Could you check a few things on this model? Use its own coordinates, in mm. Face numbers are marked on the shaded views. A direction names the side the tool comes from. Coordinates: 2 decimals unless noted, no trailing zeros. Loops run counter-clockwise (first coordinate to the right, second up) from the corner with the lowest first, then second, coordinate; pieces in that order, holes last. Notation, with made-up numbers: (72.5, -21) -> (78.5, -21) arc R18 cw to (78.5, -4) -> close; hole circle Ø10 at (37.25, 71.25). An arc over 180 degrees is marked (long way). One line per question, with ' | ' between items.
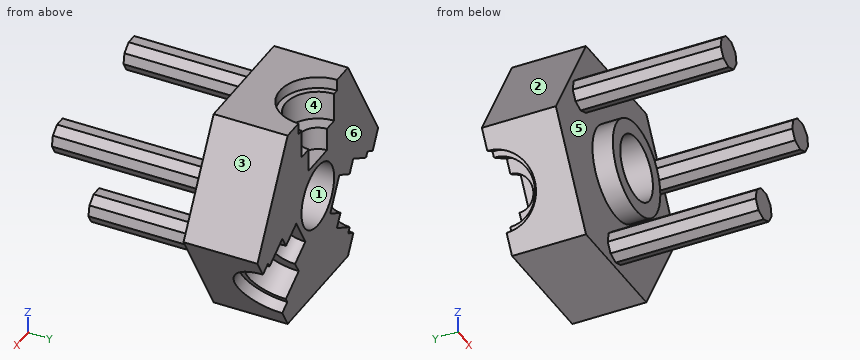
```python
from build123d import *

# Parameters (mm, degrees)
BOSS_EXTRUDE1_DEPTH = 12.7
SKETCH2_R           = 8
SKETCH2_R_2         = 5.5
BOSS_EXTRUDE2_DEPTH = 3.499999906
CIRPATTERN1_COUNT   = 3
SKETCH6_R           = 5.5
CUT_EXTRUDE1_DEPTH  = 17.199999906
BOSS_EXTRUDE3_DEPTH = 25.4


with BuildPart() as part:
    # Sketch1 → Boss-Extrude1 (new body)
    with BuildSketch(Plane(origin=(0, 0, 0), x_dir=(1, 0, 0), z_dir=(0, 1, 0))):
        Polygon((10.16, -17.597636205), (20.32, 0), (10.16, 17.597636205), (-10.16, 17.597636205), (-20.32, 0), (-10.16, -17.597636205), align=None)
    extrude(amount=BOSS_EXTRUDE1_DEPTH)

    # Sketch2 → Boss-Extrude2 (add)
    with BuildSketch(Plane.XZ):
        Circle(SKETCH2_R)
        Circle(SKETCH2_R_2, mode=Mode.SUBTRACT)
    extrude(amount=BOSS_EXTRUDE2_DEPTH)

    # Sketch5 → Cut-Revolve1 (revolve, cut)
    with BuildSketch(Plane(origin=(0, 12.7, 0), x_dir=(1, 0, 0), z_dir=(0, 1, 0))):
        Polygon((0, -17.597636205), (0, -6.597636205), (-3.065310501, -6.597636205), (-3.065310501, -10.597636205), (-5.5, -10.597636205), (-5.5, -15.597636205), (-6.5, -15.597636205), (-6.5, -17.597636205), align=None)
    cut_revolve1 = revolve(axis=Axis((0, 12.7, 17.597636205), (0, 0, -1)), mode=Mode.SUBTRACT)

    # CirPattern1: Cut-Revolve1 ×3 about axis
    cirpattern1_axis = Axis((0, 0, 0), (0, 1, 0))
    for i in range(1, CIRPATTERN1_COUNT):
        add(cut_revolve1.rotate(cirpattern1_axis, i * 360 / CIRPATTERN1_COUNT), mode=Mode.SUBTRACT)

    # Sketch6 → Cut-Extrude1 (cut, through all)
    with BuildSketch(Plane(origin=(0, 12.7, 0), x_dir=(1, 0, 0), z_dir=(0, 1, 0))):
        Circle(SKETCH6_R)
    extrude(amount=-CUT_EXTRUDE1_DEPTH, mode=Mode.SUBTRACT)

    # Sketch8 → Boss-Extrude3 (add)
    with BuildSketch(Plane(origin=(0, 0, 0), x_dir=(1, 0, 0), z_dir=(0, 1, 0))):
        Polygon((-1.915248015, 16.000954519), (-2.83973241, 14.399700576), (-2.518662349, 12.578821777), (-1.102270082, 11.390327548), (0.746698708, 11.390327548), (2.163090976, 12.578821777), (2.484161036, 14.399700576), (1.559676641, 16.000954519), (-0.177785687, 16.63333909), align=None)
        Polygon((14.814348451, -6.342126208), (13.889864056, -4.740872265), (12.152401728, -4.108487694), (10.4149394, -4.740872265), (9.490455005, -6.342126208), (9.811525066, -8.163005007), (11.227917333, -9.351499236), (13.076886123, -9.351499236), (14.49327839, -8.163005007), align=None)
        Polygon((-12.90012529, -9.658841379), (-11.0511565, -9.658841379), (-9.634764233, -8.47034715), (-9.313694172, -6.64946835), (-10.238178567, -5.048214407), (-11.975640895, -4.415829837), (-13.713103223, -5.048214407), (-14.637587618, -6.64946835), (-14.316517557, -8.47034715), align=None)
    extrude(amount=-BOSS_EXTRUDE3_DEPTH)


solid = part.part
```
Q1. Imagine slicing it at B-B on z = 13. Write out the boundary of the cut face in (x, y), plus the area to 3 significant figures.
Values follow:
outline: (-12.81, 0) -> (12.81, 0) -> (12.81, 12.7) -> (5.5, 12.7) arc R5.5 cw to (-5.5, 12.7) -> (-12.81, 12.7) -> close | area: 278 mm2
Q2. For pin 1 (4 mm diameter, centred on x = 6.5, z = 5.5, fed in from -Y); pin 2 (10 mm diameter, centred on y = 0.5, z = 14, fed in from +X); pin 3 (4.5 mm diameter, centred on x = 0.5, y = 9, fed in from +Z), each with a flat end and sliding along its axis, tell me the tip position at first contact or that it passes through.
Values follow:
pin 1: stops at y = -3.5 | pin 2: stops at x = 15.12 | pin 3: stops at z = 15.6
Q3. Please list where these lines run through material, in increasing order: L1, parallel to Z at x = 0, y = 5; L2, parallel to X at y = 8, z = 0; L3, parallel to Z at x = 0, y = 8. Write a range as [from, to].
Values follow:
L1: z = [-17.6, -5.5], [5.5, 17.6] | L2: x = [-20.32, -5.5], [5.5, 20.32] | L3: z = [-17.6, -5.5], [5.5, 10.6]
Q4. We'd pull the mould along X, two halves only. Please class the marked faces 1, 2 and 3: released by +X, released by -X, zero draft, split by the parting line, or undercut.
Values follow:
face 1: undercut | face 2: released by -X | face 3: released by +X
Q5. For the marked faces 4, 5 and 6, which set-ups out of +Z, -Z, +X, -X, +Y, -Y let a thin tool reach every point of the face, with its end or its side?
Values follow:
face 4: +Z, +Y | face 5: -Y | face 6: +Z, -Z, +X, -X, +Y
Q6. Imagine slicing it at A-A on y = -22. Write out the boundary of the cut face in (x, z).
Values follow:
outline: (-14.64, 6.65) -> (-13.71, 5.05) -> (-11.98, 4.42) -> (-10.24, 5.05) -> (-9.31, 6.65) -> (-9.63, 8.47) -> (-11.05, 9.66) -> (-12.9, 9.66) -> (-14.32, 8.47) -> close; (-2.84, -14.4) -> (-1.92, -16) -> (-0.18, -16.63) -> (1.56, -16) -> (2.48, -14.4) -> (2.16, -12.58) -> (0.75, -11.39) -> (-1.1, -11.39) -> (-2.52, -12.58) -> close; (9.49, 6.34) -> (10.41, 4.74) -> (12.15, 4.11) -> (13.89, 4.74) -> (14.81, 6.34) -> (14.49, 8.16) -> (13.08, 9.35) -> (11.23, 9.35) -> (9.81, 8.16) -> close
